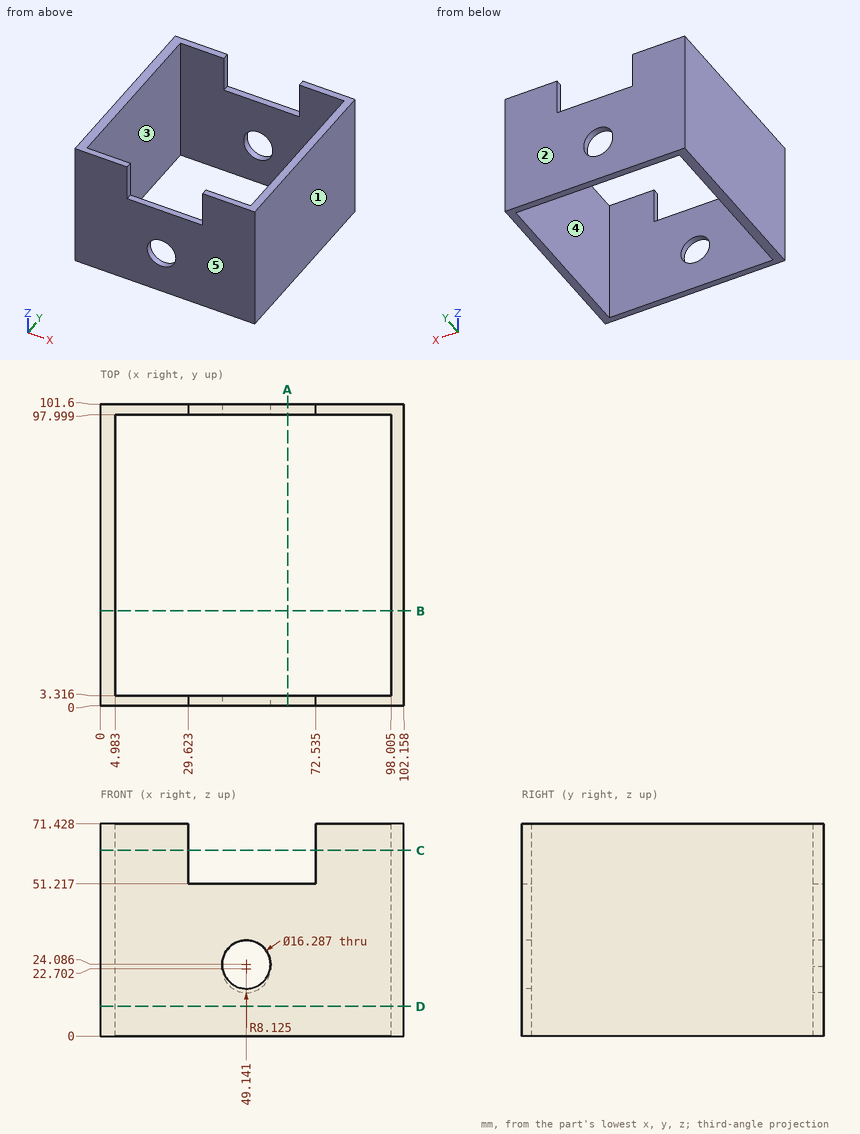
Drawing for the job (mm, zero at the part's lowest x, y, z). A direction names the side the tool comes from. Coordinates: 2 decimals unless noted, no trailing zeros. Order: outer loops, then holes, each group sorted by start corner. A loop starts at its lowest first (then second) coordinate and runs counter-clockwise, first axis right, second up.
Item 1: Band-saw the part on A-A on x = 63. List the corners of the cut face in (y, z) (1 decimal), plus the area to 3 significant figures.
Check sheet entries:
outline: (0, 0) - (3.3, 0) - (3.3, 51.2) - (0, 51.2) - close; (98, 0) - (101.6, 0) - (101.6, 51.2) - (98, 51.2) - close
area: 354 mm2
Item 2: Band-saw the part on C-C on z = 62.5. List the corners of the cut face in (x, y) (1 decimal).
Check sheet entries:
outline: (0, 0) - (29.6, 0) - (29.6, 3.3) - (5, 3.3) - (5, 98) - (29.6, 98) - (29.6, 101.6) - (0, 101.6) - close; (72.5, 0) - (102.2, 0) - (102.2, 101.6) - (72.5, 101.6) - (72.5, 98) - (98, 98) - (98, 3.3) - (72.5, 3.3) - close
Item 3: Band-saw the part on B-B on y = 32. List the corners of the cut face in (x, z) (1 decimal).
Check sheet entries:
outline: (0, 0) - (5, 0) - (5, 71.4) - (0, 71.4) - close; (98, 0) - (102.2, 0) - (102.2, 71.4) - (98, 71.4) - close
Item 4: Band-saw the part on D-D on z = 10. List the corners of the cut face in (x, y) (1 decimal).
Check sheet entries:
outline: (0, 0) - (102.2, 0) - (102.2, 101.6) - (0, 101.6) - close; hole (5, 3.3) - (98, 3.3) - (98, 98) - (5, 98) - close
Item 5: Two-plate mould, pull along Y, no slides. Class the marked faces 1, 2 and 3: +Y half, -Y half, draft (parallel to the pull), parting line (faces both ways), or undercut.
Check sheet entries:
face 1: draft
face 2: +Y half
face 3: undercut
Item 6: 3-axis set-ups, long thin cutter, end or side, ignore diameter. For the marked faces 4 and 5: which of +Z, -Z, +X, -X, +Y, -Y reach the whole face in a straight line?
Check sheet entries:
face 4: +Z, -Z
face 5: +Z, -Z, +X, -X, -Y
Item 7: Pin check, flat tips, straight feed: pin 1 Ø2.5 at (x, y) = (41, 1) entering from +Z; pin 2 Ø12 at (y, z) = (37, 10.5) entering from -X; pin 3 Ø1.5 at (x, z) = (50, 15.5) entering from +Y; pin 4 Ø10 at (x, z) = (49.14, 24.09) entering from -Y. Stop position of each tip, or through.
Check sheet entries:
pin 1: stops at z = 51.22
pin 2: stops at x = 0
pin 3: stops at y = 3.32
pin 4: passes through
Item 8: Drill centre lines: L1, parallel to X at y = 57, z = 24 (1 decimal); L2, parallel to Y at x = 92, z = 7.5 (1 decimal). Where is each one in solid material? Low to high.
Check sheet entries:
L1: x = 0 to 5, 98 to 102.2
L2: y = 0 to 3.3, 98 to 101.6
